from build123d import *

# Parameters (mm, degrees)
F1_DEPTH = 34.925
F3_DEPTH = 33.02
F4_R     = 12.7
F5_R     = 5.07999
F6_R     = 3.556
F8_DEPTH = 15.24


# Not quite as in the source:
# - a fillet or chamfer is up to 0.001 mm smaller than in the source, because OpenCascade refuses the exact size


with BuildPart() as f1:
    # F0 (on Top) → F1 (new body)
    with BuildSketch(Plane.XY):
        Polygon((9.017, 53.086), (0, 51.054), (0, -51.054), (128.219697074, -4.5338571988), (140.716, 99.822), (140.716, 111.76), (74.676, 111.76), (74.676, 68.58), (39.878, 48.006), (9.017, 48.006), align=None)
    extrude(amount=-F1_DEPTH)

    # F2 (on face) → F3 (join)
    with BuildSketch(Plane(origin=(0, 0, -34.925), x_dir=(1, 0, 0), z_dir=(0, 0, -1))):
        Polygon((-2.0574, -40.767), (0, -40.767), (0, -25.527), (-2.0574, -25.527), (-2.0574, -20.828), (-6.7564, -20.828), (-6.7564, -45.466), (-2.0574, -45.466), align=None)
        Polygon((-2.54, 39.5605), (0, 39.5605), (0, 47.1805), (-2.54, 47.1805), (-2.54, 49.276), (-4.064, 49.276), (-4.064, 37.465), (-2.54, 37.465), align=None)
        Polygon((-2.0574, -3.81), (0, -3.81), (0, 11.43), (-2.0574, 11.43), (-2.0574, 16.129), (-6.7564, 16.129), (-6.7564, -8.509), (-2.0574, -8.509), align=None)
    extrude(amount=-F3_DEPTH)

    # F4
    f4_edges = [f1.edges().sort_by_distance(p)[0] for p in [
        (39.878, 48.006, -17.4625),
        (74.676, 68.58, -17.4625),
        (128.219697, -4.533857, -17.4625),
        (140.716, 99.822, -17.4625),
    ]]
    fillet(f4_edges, radius=F4_R)

    # F5 (radius 5.08 in the source; OpenCascade refuses exactly that, so slightly less here)
    f5_edges = [f1.edges().sort_by_distance(p)[0] for p in [
        (9.017, 48.006, -17.4625),
    ]]
    fillet(f5_edges, radius=F5_R)

    # F6
    f6_edges = [f1.edges().sort_by_distance(p)[0] for p in [
        (0, 51.054, -17.4625),
    ]]
    fillet(f6_edges, radius=F6_R)

    # F7 (on face) → F8 (cut)
    with BuildSketch(Plane.XY):
        Polygon((116.3056778405, 4.923799024), (125.2853724235, 79.9126762258), (2.54, 7.34059472), (2.54, -13.589), (17.272, -31.0071923946), align=None)
    extrude(amount=-F8_DEPTH, mode=Mode.SUBTRACT)


solid = f1.part
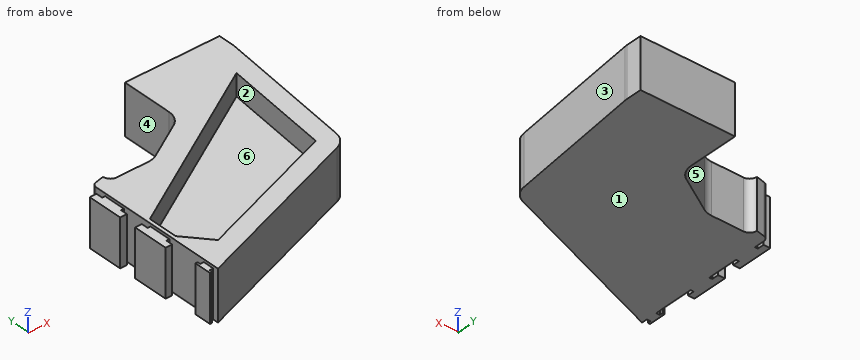
Can you work these out from the model? Positions are in its coordinate system, mm. Face numbers are marked on the shaded views. A direction names the side the tool comes from. Give positions to 0.01 mm unless a question says otherwise; leave off trailing zeros. Loops run counter-clockwise (first coordinate to the right, second up) from the corner with the lowest first, then second, coordinate; pieces in that order, holes last. Notation, with made-up numbers: (43, 7) - (76, 7) arc R19 ccw to (76, 24) - close; hole circle Ø8 at (-34.75, -20.75). An arc over 180 degrees is marked (long way). Answer as a JSON object with one key per item and string values.
Q1. Will these pins go through, and if not, where does the flat tip stop? P1, Ø2.5, axis at y = 6, z = -19, coming from the +X side; P2, Ø2, axis at x = -2, y = -45, coming from the +Z side (3 decimals); P3, Ø2.5, axis at x = -4, z = -26.5, coming from the +Y side; P4, Ø2.5, axis at x = -1, z = -24.5, coming from the -Y side.
Geometry says:
{"P1": "x = 129.63", "P2": "z = -1.905", "P3": "y = 45.47", "P4": "y = -51.05"}
Q2. Imagine slicing it at B-B on x = 77. Write out the boundary of the cut face in (y, z) (3 decimals), plus the area to 3 significant figures.
Geometry says:
{"outline": "(-23.117, -34.925) - (111.76, -34.925) - (111.76, 0) - (51.364, 0) - (51.364, -15.24) - (-9.337, -15.24) - (-9.337, 0) - (-23.117, 0) - close", "area": "3,790 mm²"}
Q3. Imagine slicing it at C-C on y = -21. Write out the boundary of the cut face in (x, z) (3 decimals), plus the area to 3 significant figures.
Geometry says:
{"outline": "(0, -34.925) - (82.835, -34.925) - (82.835, 0) - (44.854, 0) - (44.854, -15.24) - (8.808, -15.24) - (8.808, 0) - (0, 0) - close", "area": "2,340 mm²"}
Q4. Imagine slicing it at D-D on y = 1. Write out the boundary of the cut face in (x, z) (3 decimals), plus the area to 3 significant figures.
Geometry says:
{"outline": "(-6.756, -34.925) - (128.677, -34.925) - (128.677, 0) - (105.491, 0) - (105.491, -15.24) - (2.54, -15.24) - (2.54, 0) - (0, 0) - (0, -1.905) - (-6.756, -1.905) - close", "area": "3,150 mm²"}
Q5. Imagine slicing it at A-A on y = 43.5. Write out the boundary of the cut face in (x, z) (1 decimal), plus the area to 3 significant figures.
Geometry says:
{"outline": "(-6.8, -34.9) - (-2.1, -34.9) - (-2.1, -1.9) - (-6.8, -1.9) - close; (0, -34.9) - (134, -34.9) - (134, 0) - (120.9, 0) - (120.9, -15.2) - (63.7, -15.2) - (63.7, 0) - (0, 0) - close", "area": "3,960 mm²"}
Q6. If we mould it in two halves opening along Y, with no side actions, what happens to the marked faces 1, 2 and 3? For each: pulls with the +Y half, pulls with the -Y half, needs draft (parallel to the pull), parting line crosses it, or undercut.
Geometry says:
{"face 1": "needs draft", "face 2": "undercut", "face 3": "pulls with the -Y half"}
Q7. Which directions (+Z, -Z, +X, -X, +Y, -Y) give clear straight access to the entire face, cutting with the end or side of a thin tool? Please do the marked faces 4, 5 and 6.
Geometry says:
{"face 4": "+Z, -Z, -X, +Y", "face 5": "+Z, -Z, +Y", "face 6": "+Z"}
Q8. If I drill on L1, parallel to X at y = 43.5, z = -11; L2, parallel to Z at x = 45, y = -5.5 (3 decimals); L3, parallel to X at y = 43, z = -26.5, over which ranges is the centre line in solid material (lowest first)?
Geometry says:
{"L1": "-6.76 to -2.06, 0 to 63.7, 120.93 to 133.97", "L2": "-34.925 to -15.24", "L3": "-6.76 to -2.06, 0 to 133.91"}
